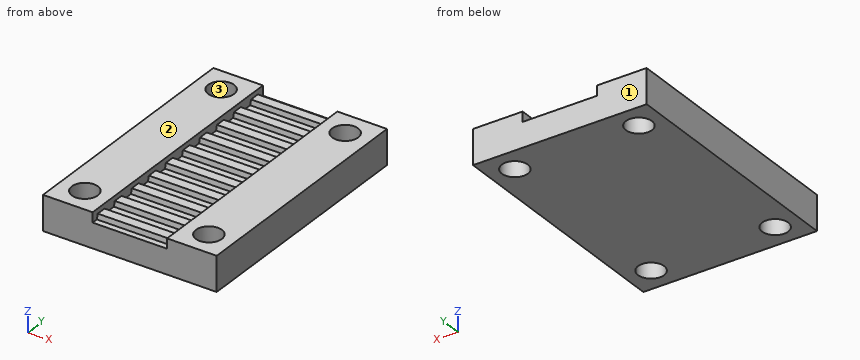
from build123d import *

# Parameters (mm, degrees)
SKETCH_W     = 15
SKETCH_H     = 50
PAD_DEPTH    = 5
PAD001_DEPTH = 15
SKETCH002_W  = 10
SKETCH002_H  = 50
PAD002_DEPTH = 7
SKETCH003_W  = 10
SKETCH003_H  = 50
PAD003_DEPTH = 7
SKETCH004_R  = 2.625
POCKET_DEPTH = 7


with BuildPart() as part:
    # Sketch → Pad (new body)
    with BuildSketch(Plane.XY):
        Rectangle(SKETCH_W, SKETCH_H)
    extrude(amount=PAD_DEPTH)

    # Sketch001 (on Face3 of Pad) → Pad001 (join)
    with BuildSketch(Plane.YZ.offset(7.5)):
        Polygon((-23.75, 5), (-23.5, 6), (-21.5, 6), (-21.25, 5), align=None)
        Polygon((-18.75, 5), (-18.5, 6), (-16.5, 6), (-16.25, 5), align=None)
        Polygon((-13.75, 5), (-13.5, 6), (-11.5, 6), (-11.25, 5), align=None)
        Polygon((-8.75, 5), (-8.5, 6), (-6.5, 6), (-6.25, 5), align=None)
        Polygon((-3.75, 5), (-3.5, 6), (-1.5, 6), (-1.25, 5), align=None)
        Polygon((1.25, 5), (1.5, 6), (3.5, 6), (3.75, 5), align=None)
        Polygon((6.25, 5), (6.5, 6), (8.5, 6), (8.75, 5), align=None)
        Polygon((11.25, 5), (11.5, 6), (13.5, 6), (13.75, 5), align=None)
        Polygon((16.25, 5), (16.5, 6), (18.5, 6), (18.75, 5), align=None)
        Polygon((21.25, 5), (21.5, 6), (23.5, 6), (23.75, 5), align=None)
    extrude(amount=-PAD001_DEPTH)

    # Sketch002 (on Face4 of Pad001) → Pad002 (join)
    with BuildSketch(Plane(origin=(0, 0, 0), x_dir=(1, 0, 0), z_dir=(0, 0, -1))):
        with Locations((12.5, 0)):
            Rectangle(SKETCH002_W, SKETCH002_H)
    extrude(amount=-PAD002_DEPTH)

    # Sketch003 (on Face4 of Pad002) → Pad003 (join)
    with BuildSketch(Plane(origin=(0, 0, 0), x_dir=(1, 0, 0), z_dir=(0, 0, -1))):
        with Locations((-12.5, 0)):
            Rectangle(SKETCH003_W, SKETCH003_H)
    extrude(amount=-PAD003_DEPTH)

    # Sketch004 (on Face12 of Pad003) → Pocket (cut)
    with BuildSketch(Plane(origin=(0, 0, 0), x_dir=(1, 0, 0), z_dir=(0, 0, -1))):
        with Locations((-12.5, 20)):
            Circle(SKETCH004_R)
        with Locations((-12.5, -20)):
            Circle(SKETCH004_R)
        with Locations((12.5, -20)):
            Circle(SKETCH004_R)
        with Locations((12.5, 20)):
            Circle(SKETCH004_R)
    extrude(amount=-POCKET_DEPTH, mode=Mode.SUBTRACT)


solid = part.part
Could you check a few things on this model? Use its own coordinates, in mm. Face numbers are marked on the shaded views. Give positions to 0.01 mm unless a question says otherwise; leave off trailing zeros. Order: outer loops, then holes, each group sorted by start corner. A loop starts at its lowest first (then second) coordinate and runs counter-clockwise, first axis right, second up. Notation, with made-up numbers: (68.25, 36.5) -> (124.25, 36.5) arc R22 cw to (124.25, 59.5) -> close; hole circle Ø5 at (77.25, 44.5). An arc over 180 degrees is marked (long way). Answer in a Markdown table with one row per item. Add a question column.
Item 1: Imagine slicing it at A-A (y = 20). List the corners of the cut face in (x, z) for me (3 decimals), and give its area (4 significant figures).
Item 2: Imagine slicing it at D-D (y = -2.5). List the corners of the cut face in (x, z) for me, and give its area (3 significant figures).
Item 3: We'd pull the mould along Y, two halves only. Please class the marked faces 1, 2 and 3: pulls with the +Y half, pulls with the -Y half, needs draft (parallel to the pull), parting line crosses it, or undercut.
Item 4: Please list where these lines run through material, in increasing order: probe 1 along Y at (x, z) = (-12.5, 4.5) (3 decimals); probe 2 along X at (y, z) = (-20, 4) (3 decimals); probe 3 along X at (y, z) = (1, 6.75).
Item 5: I'm going to push flat-ended pins straight in: P1, Ø0.8, axis at x = -0.5, y = 9.5, coming from the +Z side; P2, Ø0.6, axis at x = -3, y = 7, coming from the +Z side; P3, Ø3, axis at x = -12.5, y = -20, coming from the +Z side. Where does each tip first touch, or does it pass through?
Item 6: Imagine slicing it at B-B (x = -12.5). List the corners of the cut face in (y, z) for me (3 decimals), and give its area (4 significant figures).
Result:
| question | item | result |
|---|---|---|
| 1 | outline | (-17.5, 0) -> (-15.125, 0) -> (-15.125, 7) -> (-17.5, 7) -> close; (-9.875, 0) -> (9.875, 0) -> (9.875, 7) -> (7.5, 7) -> (7.5, 5) -> (-7.5, 5) -> (-7.5, 7) -> (-9.875, 7) -> close; (15.125, 0) -> (17.5, 0) -> (17.5, 7) -> (15.125, 7) -> close |
| 1 | area | 141.5 mm2 |
| 2 | outline | (-17.5, 0) -> (17.5, 0) -> (17.5, 7) -> (7.5, 7) -> (7.5, 6) -> (-7.5, 6) -> (-7.5, 7) -> (-17.5, 7) -> close |
| 2 | area | 230 mm2 |
| 3 | face 1 | pulls with the +Y half |
| 3 | face 2 | needs draft |
| 3 | face 3 | undercut |
| 4 | probe 1 | -25 to -22.625, -17.375 to 17.375, 22.625 to 25 |
| 4 | probe 2 | -17.5 to -15.125, -9.875 to 9.875, 15.125 to 17.5 |
| 4 | probe 3 | -17.5 to -7.5, 7.5 to 17.5 |
| 5 | P1 | z = 5 |
| 5 | P2 | z = 6 |
| 5 | P3 | through |
| 6 | outline | (-25, 0) -> (-22.625, 0) -> (-22.625, 7) -> (-25, 7) -> close; (-17.375, 0) -> (17.375, 0) -> (17.375, 7) -> (-17.375, 7) -> close; (22.625, 0) -> (25, 0) -> (25, 7) -> (22.625, 7) -> close |
| 6 | area | 276.5 mm2 |
